Design review of the part built by this model. Coordinates are the model's own, in mm. A direction names the side the tool comes from. Coordinates: 2 decimals unless noted, no trailing zeros. Loops run counter-clockwise (first coordinate to the right, second up) from the corner with the lowest first, then second, coordinate; pieces in that order, holes last. Notation, with made-up numbers: M 22.5,4.5 L 73.5,4.5 A31 cw 73.5,39.5 Z; hole C 1.25,44.5 d10. An arc over 180 degrees is marked long. One line per item, written item: value.
Autodesk Inventor part; units mm, degrees
ref_plane "YZ Plane" through (0, 0, 0) normal (1, 0, 0) x (0, 1, 0)
ref_plane "XZ Plane" through (0, 0, 0) normal (0, 1, 0) x (-1, 0, 0)
ref_plane "XY Plane" through (0, 0, 0) normal (0, 0, 1) x (1, 0, 0)
sketch "Szkic1" plane through (0, 0, 0) normal (0, 1, 0) x (-1, 0, 0)
  circle A0 centre (0, 0) radius 1.75
  line L0 (18.5, 10) -> (-21.5, 10)
  line L1 (-21.5, 10) -> (-21.5, -10)
  line L2 (-21.5, -10) -> (18.5, -10)
  line L3 (18.5, -10) -> (18.5, 10)
  line L4 (-19.5, 9) -> (16.5, 9)
  line L5 (16.5, 9) -> (16.5, -9)
  line L6 (16.5, -9) -> (-19.5, -9)
  line L7 (-19.5, -9) -> (-19.5, 9)
  dimension "d0" = 3.5
  dimension "d1" = 20
  dimension "d2" = 40
  dimension "d3" = 36
  dimension "d4" = 18
  dimension "d9" = 16.5
  dimension "d10" = 2
extrude "Wyciągnięcie proste1" add sketch "Szkic1" along normal blind 6 contours L3 L2 L1 L0
extrude "Wyciągnięcie proste2" add sketch "Szkic1" along normal blind 1 and the other way blind 2 contours L3 L2 L1 L0 | L4 L5 L6 L7
sketch "Szkic2" plane through (21.5, 0, 10) normal (1, 0, 0) x (0, 0, -1)
  line L0 (10, 0) -> (10, 3.2)
  line L1 (10, 0) -> (13.2, 0) construction
  line L2 (6.5, 3.2) -> (13.5, 3.2) construction
  line L3 (6.5, 1.7) -> (13.5, 1.7)
  line L4 (13.5, 4.7) -> (6.5, 4.7)
  arc A0 (6.5, 4.7) -> (6.5, 1.7) centre (6.5, 3.2) ccw
  arc A1 (13.5, 1.7) -> (13.5, 4.7) centre (13.5, 3.2) ccw
  dimension "d11" = 3.2
  dimension "d12" = 90
  dimension "d13" = 3.5
  dimension "d14" = 3
extrude "Wyciągnięcie proste3" cut sketch "Szkic2" against normal blind 10
sketch "Szkic3" plane through (-18.5, 0, -10) normal (-1, 0, 0) x (0, 0, 1)
  line L0 (10, 0) -> (10, 2.5)
  line L1 (10, 0) -> (12.5, 0) construction
  line L2 (5.25, 4.5) -> (14.75, 4.5)
  line L3 (14.75, 4.5) -> (14.75, 0.5)
  line L4 (14.75, 0.5) -> (5.25, 0.5)
  line L5 (5.25, 0.5) -> (5.25, 4.5)
  line L6 (5.25, 4.5) -> (14.75, 0.5) construction
  line L7 (14.75, 4.5) -> (5.25, 0.5) construction
  dimension "d17" = 2.5
  dimension "d18" = 90
  dimension "d19" = 9.5
  dimension "d20" = 4
extrude "Wyciągnięcie proste4" cut sketch "Szkic3" against normal blind 10
sketch "Szkic4" plane through (0, 1, 0) normal (0, 1, 0) x (1, 0, 0)
  circle A0 centre (0, 0) radius 1.75
  circle A1 centre (0, 0) radius 3.5
  dimension "d23" = 7
extrude "Wyciągnięcie proste5" cut sketch "Szkic4" against normal blind 2
sketch "Szkic5" plane through (-18.5, 6, 10) normal (0, 0, 1) x (1, 0, 0)
  line L0 (2, -5) -> (2, 0)
  line L1 (2, -5) -> (2, 0)
  line L2 (2, 0) -> (2, -5)
  line L3 (2, -5) -> (2, -5.5)
  line L4 (0, -5.5) -> (10, -5.5)
  line L5 (2, -5.5) -> (7, -5.5)
  circle A0 centre (4.5, -3) radius 2.5
  point P0 (18.5, -6)
  dimension "d28" = 5
  dimension "d29" = 5
  dimension "d32" = 2.5
  dimension "d33" = 2.5
extrude "Wyciągnięcie proste6" cut sketch "Szkic5" against normal blind 10 contours A0
properties part number "elektronika"
(1) We need section C-C on x = 9.5. State the section outline as (y, z) points.
Reply:
outline: M -2,-10 L 6,-10 L 6,-9 L 1,-9 L 1,9 L 6,9 L 6,10 L -2,10 Z
(2) We need section B-B on z = 0. State the section outline as (x, y) points, then the cut area to 4 significant figures.
Reply:
outline: M -18.5,-2 L -1.75,-2 L -1.75,-1 L -3.5,-1 L -3.5,1 L -8.5,1 L -8.5,0.5 L -18.5,0.5 Z; M -18.5,4.5 L -16.5,4.5 L -16.5,6 L -18.5,6 Z; M 1.75,-2 L 21.5,-2 L 21.5,1.7 L 19.5,1.7 L 19.5,1 L 3.5,1 L 3.5,-1 L 1.75,-1 Z; M 19.5,4.7 L 21.5,4.7 L 21.5,6 L 19.5,6 Z
area: 104.5 mm2
(3) Mouldability with a two-part tool opening along Z and no side actions: class faces 1 (the flat face through (-14, 0.5, 0)), 2 (the flat face through (-18.5, 0, 0)), 3 (the flat face through (1, 2, 10)) as released by +Z, released by -Z, zero draft, split by the parting line, or undercut.
Reply:
face 1: undercut
face 2: zero draft
face 3: released by +Z
(4) Tool access review of faces 4 (the cylindrical face through (20.5, 3.2, 5)), 5 (the flat face through (21, 1.7, 0)), 6 (the cylindrical face through (3.233, 0.014, 1.341)), 7 (the flat face through (-17, 2, -4.75)), 8 (the cylindrical face through (-12.85, 0.78, 8.58)): name each direction out of +Z, -Z, +X, -X, +Y, -Y from which nothing blocks a thin tool from reaching the whole face with its end or side.
Reply:
face 4: +X
face 5: +X, -X
face 6: +Y
face 7: -X
face 8: +Z
(5) Insertion check: pin 1 (1.5 mm diameter, centred on y = 4, z = -2, fed in from -X); pin 2 (5.5 mm diameter, centred on x = 0, z = 0, fed in from +Y); pin 3 (1 mm diameter, centred on x = 13.5, z = 6.5, fed in from +Y). Each pin has a flat end and moves straight along its axis. Give the tip position at first contact, or say it passes through.
Reply:
pin 1: stops at x = -18.5
pin 2: stops at y = -1
pin 3: stops at y = 1
(6) We need section D-D on z = -8. State the section outline as (x, y) points, then the cut area to 3 significant figures.
Reply:
outline: M -18.5,-2 L 21.5,-2 L 21.5,6 L 19.5,6 L 19.5,1 L -16.5,1 L -16.5,6 L -18.5,6 Z
area: 140 mm2
(7) We need section A-A on x = 0. State the section outline as (y, z) points.
Reply:
outline: M -2,-10 L 6,-10 L 6,-9 L 1,-9 L 1,-3.5 L -1,-3.5 L -1,-1.75 L -2,-1.75 Z; M -2,1.75 L -1,1.75 L -1,3.5 L 1,3.5 L 1,9 L 6,9 L 6,10 L -2,10 Z
(8) To check wall thickness, follow line 1 along X through (y, z) = (0.45, 0); line 2 along Z through (x, y) = (-9, 2); line 3 along X through (y, z) = (4.25, -5). State the ranges of each line that lie inside material, in increasing order. Write a range as [from, to].
Reply:
line 1: x = [-18.5, -3.5], [3.5, 21.5]
line 2: z = [-10, -9], [9, 10]
line 3: x = [-18.5, -16.5], [19.5, 21.5]
